The listing builds one solid part. Answer for the finished solid, in the listing's coordinates (mm). A direction names the side the tool comes from. Coordinates: 2 decimals unless noted, no trailing zeros. Order: outer loops, then holes, each group sorted by start corner. A loop starts at its lowest first (then second) coordinate and runs counter-clockwise, first axis right, second up. Notation, with made-up numbers: (-34.75, 59.25) - (6.25, 59.25) arc R21 cw to (6.25, 78.25) - close; hole circle Ø5 at (37, 19). An arc over 180 degrees is marked (long way). Use a Markdown table: item, result. Add a question column.
Item 1: The part is cut by section A-A, the plane y = 38. Give the vertices of the cut face in (x, z).
Item 2: For faces 1 (the flat face through (48, 50.5, -84)), 2 (the flat face through (-53, 35, 12)), 3 (the flat face through (53, 2, -62.5)), determine the directions among +Z, -Z, +X, -X, +Y, -Y from which every point of the face is accessible in a straight line to the end or side of a thin tool.
Item 3: The mould has two halves that part along Z. Classify faces 4 (the flat face through (53, 2, 62.5)), 5 (the flat face through (1, 36, 59.5)), 6 (the flat face through (45.5, 35, -13)): released by +Z, released by -Z, zero draft, split by the parting line, or undercut.
Item 4: The part is cut by section C-C, the plane z = 37.5. Give the vertices of the cut face in (x, y), then the cut area to 3 significant figures.
Item 5: Flat-ended cylindrical pins translate along their axes: P1, Ø5, axis at y = 24.5, z = -18.5, coming from the +X side; P2, Ø4, axis at x = -53.5, y = 2, coming from the -Z side; P3, Ø8, axis at x = 56.5, z = -68.5, coming from the +Y side. Find the tip coordinate at first contact, or state that the pin passes through.
Item 6: The part is cut by section B-B, the plane x = 10. Give the vertices of the cut face in (y, z), then the cut area to 3 significant figures.
Item 7: Find the intervals of material crossed by line 1 along X through (y, z) = (3.85, 67.5); line 2 along X through (y, z) = (31, -54); line 3 along X through (y, z) = (2, -67), in increasing order.
from build123d import *

# Parameters (mm, degrees)
SKETCH2_W                = 100
SKETCH2_H                = 145
BOSS_EXTRUDE1_DEPTH      = 75
SKETCH3_W                = 91
SKETCH3_H                = 140
CUT_EXTRUDE1_DEPTH       = 71
BOSS_EXTRUDE2_DEPTH      = 5
M3_CLEARANCE_HOLE2_D     = 3.2
M3_CLEARANCE_HOLE2_DEPTH = 12
M3_CLEARANCE_HOLE2_TIP   = 0.96137699
SKETCH11_W               = 8
SKETCH11_H               = 30
SKETCH11_W_2             = 2
SKETCH11_H_2             = 21
BOSS_EXTRUDE4_DEPTH      = 4
SKETCH13_W               = 91
SKETCH13_H               = 71
BOSS_EXTRUDE6_DEPTH      = 8
BOSS_EXTRUDE7_DEPTH      = 8
SKETCH12_W               = 8
SKETCH12_H               = 30
SKETCH12_W_2             = 2
SKETCH12_H_2             = 21
BOSS_EXTRUDE5_DEPTH      = 4.5
FILLET1_R                = 2


with BuildPart() as part:
    # Sketch2 → Boss-Extrude1 (new body)
    with BuildSketch(Plane(origin=(0, 0, 0), x_dir=(1, 0, 0), z_dir=(0, 1, 0))):
        Rectangle(SKETCH2_W, SKETCH2_H)
    extrude(amount=BOSS_EXTRUDE1_DEPTH)

    # Sketch3 → Cut-Extrude1 (cut)
    with BuildSketch(Plane.XZ):
        with Locations((0, -2.5)):
            Rectangle(SKETCH3_W, SKETCH3_H)
    extrude(amount=-CUT_EXTRUDE1_DEPTH, mode=Mode.SUBTRACT)

    # Sketch4 → Boss-Extrude2 (add)
    with BuildSketch(Plane.XZ):
        with BuildLine():
            Line((-50, 72.5), (-55, 72.5))
            ThreePointArc((-55, 72.5), (-60, 67.5), (-55, 62.5))
            Line((-55, 62.5), (-50, 62.5))
            Line((-50, 62.5), (-50, 72.5))
        make_face()
        with BuildLine():
            Line((50, 72.5), (55, 72.5))
            ThreePointArc((55, 72.5), (60, 67.5), (55, 62.5))
            Line((55, 62.5), (50, 62.5))
            Line((50, 62.5), (50, 72.5))
        make_face()
        with BuildLine():
            Line((-50, -72.5), (-55, -72.5))
            ThreePointArc((-55, -72.5), (-60, -67.5), (-55, -62.5))
            Line((-55, -62.5), (-50, -62.5))
            Line((-50, -62.5), (-50, -72.5))
        make_face()
        with BuildLine():
            Line((50, -72.5), (55, -72.5))
            ThreePointArc((55, -72.5), (60, -67.5), (55, -62.5))
            Line((55, -62.5), (50, -62.5))
            Line((50, -62.5), (50, -72.5))
        make_face()
    extrude(amount=-BOSS_EXTRUDE2_DEPTH)

    # M3 Clearance Hole2
    with Locations(Plane(origin=(0, 5, 0), x_dir=(1, 0, 0), z_dir=(0, 1, 0))):
        with Locations((-55, 67.5), (55, 67.5), (55, -67.5), (-55, -67.5)):
            Hole(M3_CLEARANCE_HOLE2_D / 2, depth=M3_CLEARANCE_HOLE2_DEPTH)
            with Locations((0, 0, -(M3_CLEARANCE_HOLE2_DEPTH + M3_CLEARANCE_HOLE2_TIP / 2))):  # 118° drill point
                Cone(0, M3_CLEARANCE_HOLE2_D / 2, M3_CLEARANCE_HOLE2_TIP, mode=Mode.SUBTRACT)

    # Sketch11 → Boss-Extrude4 (add, symmetric)
    with BuildSketch(Plane(origin=(0, 0, 12.5), x_dir=(-1, 0, 0), z_dir=(0, 0, -1))):
        with Locations((54, 35.5)):
            Rectangle(SKETCH11_W, SKETCH11_H)
        with Locations((54, 35.5)):
            Rectangle(SKETCH11_W_2, SKETCH11_H_2, mode=Mode.SUBTRACT)
    extrude(amount=BOSS_EXTRUDE4_DEPTH, both=True)

    # Sketch13 → Boss-Extrude6 (add)
    with BuildSketch(Plane(origin=(0, 0, 67.5), x_dir=(-1, 0, 0), z_dir=(0, 0, -1))):
        with Locations((0, 35.5)):
            Rectangle(SKETCH13_W, SKETCH13_H)
    extrude(amount=BOSS_EXTRUDE6_DEPTH)

    # Sketch15 → Boss-Extrude7 (add)
    with BuildSketch(Plane(origin=(0, 0, -72.5), x_dir=(-1, 0, 0), z_dir=(0, 0, -1))):
        Polygon((-50, 5), (-50, 0), (-45.5, 0), (-45.5, 71), (45.5, 71), (45.5, 0), (50, 0), (50, 5), (50, 75), (-50, 75), align=None)
    extrude(amount=BOSS_EXTRUDE7_DEPTH)

    # Sketch12 → Boss-Extrude5 (add)
    with BuildSketch(Plane(origin=(50, 0, 0), x_dir=(0, 0, -1), z_dir=(1, 0, 0))):
        with Locations((84.5, 35.5)):
            Rectangle(SKETCH12_W, SKETCH12_H)
        with Locations((84.5, 35.5)):
            Rectangle(SKETCH12_W_2, SKETCH12_H_2, mode=Mode.SUBTRACT)
    extrude(amount=-BOSS_EXTRUDE5_DEPTH)

    # Fillet1
    fillet1_edges = [part.edges().sort_by_distance(p)[0] for p in [
        (-50, 50.5, 12.5),
        (-50, 20.5, 12.5),
        (-58, 20.5, 12.5),
        (-58, 50.5, 12.5),
        (-50, 75, -4),
        (-50, 2.5, -72.5),
        (50, 2.5, -72.5),
        (0, 75, 72.5),
        (47.75, 20.5, -88.5),
        (47.75, 50.5, -88.5),
        (47.75, 50.5, -80.5),
        (47.75, 20.5, -80.5),
        (50, 75, -4),
        (50, 40, 72.5),
        (-50, 40, 72.5),
    ]]
    fillet(fillet1_edges, radius=FILLET1_R)


solid = part.part
Solution:
| question | item | result |
|---|---|---|
| 1 | outline | (-58, 8.5) - (-55, 8.5) - (-55, 16.5) - (-58, 16.5) - close; (-53, 8.5) - (-50, 8.5) - (-50, -80.5) - (-45.5, -80.5) - (-45.5, 59.5) - (45.5, 59.5) - (45.5, -83.5) - (50, -83.5) - (50, 70.5) arc R2 ccw to (48, 72.5) - (-48, 72.5) arc R2 ccw to (-50, 70.5) - (-50, 16.5) - (-53, 16.5) - close; (45.5, -88.5) - (50, -88.5) - (50, -85.5) - (45.5, -85.5) - close |
| 2 | face 1 | -Z, +X, -X, +Y |
| 2 | face 2 | +Z, -Z |
| 2 | face 3 | +X, +Y, -Y |
| 3 | face 4 | undercut |
| 3 | face 5 | released by -Z |
| 3 | face 6 | zero draft |
| 4 | outline | (-50, 0) - (-45.5, 0) - (-45.5, 71) - (45.5, 71) - (45.5, 0) - (50, 0) - (50, 73) arc R2 ccw to (48, 75) - (-48, 75) arc R2 ccw to (-50, 73) - close |
| 4 | area | 1,040 mm2 |
| 5 | P1 | stops at x = 50 |
| 5 | P2 | stops at z = -72.56 |
| 5 | P3 | stops at y = 5 |
| 6 | outline | (0, 59.5) - (71, 59.5) - (71, -80.5) - (75, -80.5) - (75, 70.5) arc R2 ccw to (73, 72.5) - (0, 72.5) - close |
| 6 | area | 1,530 mm2 |
| 7 | line 1 | x = -60 to -56.6, -53.4 to 53.4, 56.6 to 60 |
| 7 | line 2 | x = -50 to -45.5, 45.5 to 50 |
| 7 | line 3 | x = -59.97 to -56.52, -53.48 to -45.5, 45.5 to 53.48, 56.52 to 59.97 |
